Input: part model. Units: mm. Frame: model coordinates. Face numbers are marked on the shaded views. A direction names the side the tool comes from. Round coordinates to 2 decimals unless told otherwise and drop trailing zeros. Order: outer loops, then holes, each group sorted by start corner. A loop starts at its lowest first (then second) coordinate and runs counter-clockwise, first axis right, second up. Notation, with made-up numbers: (-29, 41) -> (10, 41) arc R20 cw to (10, 60) -> close; hole circle Ø11 at (-35, -20). An arc over 180 degrees is marked (long way). Answer as CSV lines item,"result". Start each with the question number.
1) Section query D-D, the plane y = -3.5. Output: boundary loops of the cut face in (x, z), and give its area (3 significant figures).
2) Line query: L1, parallel to Y at x = 10, z = 3.35; L2, parallel to X at y = 3.5, z = 3.25; L3, parallel to Y at x = 90.5, z = 1.5. Output: solid intervals per line, ascending.
3) Section query C-C, the plane z = 3.25. Output: boundary loops of the cut face in (x, y).
4) Section query B-B, the plane x = 10. Output: boundary loops of the cut face in (y, z).
5) Section query A-A, the plane y = 5. Output: boundary loops of the cut face in (x, z), and give its area (3 significant figures).
6) First-contact query: P1, Ø1, axis at y = 3.5, z = 3.5, coming from the +X side; P2, Ø1, axis at x = 36.5, z = 6, coming from the +Y side; P3, Ø1.6, axis at y = -1.5, z = 8.5, coming from the -X side; P4, Ø5, axis at x = 25, y = 5, coming from the +Z side. Flat tips, straight axial feed; report the tip coordinate or a pass-through.
7) Access query for the marked faces 1, 2 and 3. Directions: +Z, -Z, +X, -X, +Y, -Y. A direction counts if a zero-diameter tool reaches every point of the face in a straight line with its end or side. Return the directions, or none.
```python
from build123d import *

# Parameters (mm, degrees)
SKETCH_1_W          = 100
SKETCH_1_H          = 25
EXTRUDE_1_DEPTH     = 5
SKETCH_2_W          = 53
SKETCH_2_H          = 5
EXTRUDE_2_DEPTH     = 5
SKETCH_5_W          = 56
SKETCH_5_H          = 5
CUT_EXTRUDE_1_DEPTH = 10
SKETCH_6_W          = 5
SKETCH_6_H          = 5
EXTRUDE_3_DEPTH     = 47
SKETCH_7_W          = 56
SKETCH_7_H          = 5
CUT_EXTRUDE_2_DEPTH = 14.5
SKETCH_8_W          = 53
SKETCH_8_H          = 5.5
EXTRUDE_4_DEPTH     = 5.95
SKETCH_9_W          = 10.95
SKETCH_9_H          = 5.5
EXTRUDE_5_DEPTH     = 32.46
SKETCH_11_W         = 44
SKETCH_11_H         = 5
CUT_EXTRUDE_3_DEPTH = 15
SKETCH_12_R         = 2.25
CUT_EXTRUDE_4_DEPTH = 15


with BuildPart() as part:
    # 草图1 → 凸台-拉伸1 (new body)
    with BuildSketch(Plane.XY):
        with Locations((50, 12.5)):
            Rectangle(SKETCH_1_W, SKETCH_1_H)
    extrude(amount=EXTRUDE_1_DEPTH)

    # 草图2 → 凸台-拉伸2 (add)
    with BuildSketch(Plane.XZ):
        with Locations((73.5, 2.5)):
            Rectangle(SKETCH_2_W, SKETCH_2_H)
    extrude(amount=EXTRUDE_2_DEPTH)

    # 草图5 → 切除-拉伸1 (cut)
    with BuildSketch(Plane(origin=(0, 25, 0), x_dir=(1, 0, 0), z_dir=(0, 1, 0))):
        with Locations((72, -2.5)):
            Rectangle(SKETCH_5_W, SKETCH_5_H)
    extrude(amount=-CUT_EXTRUDE_1_DEPTH, mode=Mode.SUBTRACT)

    # 草图6 → 凸台-拉伸3 (add)
    with BuildSketch(Plane.ZY.offset(-47)):
        with Locations((2.5, -2.5)):
            Rectangle(SKETCH_6_W, SKETCH_6_H)
    extrude(amount=EXTRUDE_3_DEPTH)

    # 草图7 → 切除-拉伸2 (cut)
    with BuildSketch(Plane(origin=(0, 15, 0), x_dir=(1, 0, 0), z_dir=(0, 1, 0))):
        with Locations((72, -2.5)):
            Rectangle(SKETCH_7_W, SKETCH_7_H)
    extrude(amount=-CUT_EXTRUDE_2_DEPTH, mode=Mode.SUBTRACT)

    # 草图8 → 凸台-拉伸4 (add)
    with BuildSketch(Plane.XY.offset(5)):
        with Locations((73.5, -2.25)):
            Rectangle(SKETCH_8_W, SKETCH_8_H)
    extrude(amount=EXTRUDE_4_DEPTH)

    # 草图9 → 凸台-拉伸5 (add)
    with BuildSketch(Plane(origin=(100, 0, 0), x_dir=(0, 0, -1), z_dir=(1, 0, 0))):
        with Locations((-5.475, -2.25)):
            Rectangle(SKETCH_9_W, SKETCH_9_H)
    extrude(amount=EXTRUDE_5_DEPTH)

    # 草图11 → 切除-拉伸3 (cut)
    with BuildSketch(Plane(origin=(0, 25, 0), x_dir=(1, 0, 0), z_dir=(0, 1, 0))):
        with Locations((22, -2.5)):
            Rectangle(SKETCH_11_W, SKETCH_11_H)
    extrude(amount=-CUT_EXTRUDE_3_DEPTH, mode=Mode.SUBTRACT)

    # 草图12 → 切除-拉伸4 (cut)
    with BuildSketch(Plane(origin=(0, 0, 0), x_dir=(-1, 0, 0), z_dir=(0, 0, -1))):
        with Locations((-10, 5)):
            Circle(SKETCH_12_R)
        with Locations((-25, 5)):
            Circle(SKETCH_12_R)
    extrude(amount=-CUT_EXTRUDE_4_DEPTH, mode=Mode.SUBTRACT)


solid = part.part
```
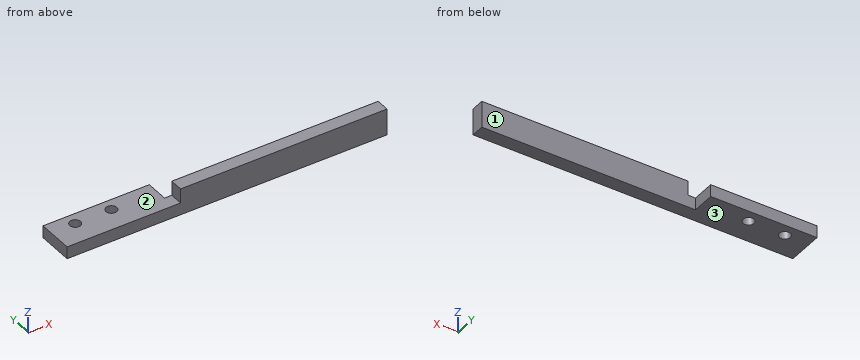
Findings:
1,outline,"(0, 0) -> (132.46, 0) -> (132.46, 10.95) -> (47, 10.95) -> (47, 5) -> (0, 5) -> close"
1,area,"1,170 mm^2"
2,L1,"y = -5 to 2.75, 7.25 to 10"
2,L2,"x = 0 to 8.32, 11.68 to 23.32, 26.68 to 44"
2,L3,"y = -5 to 0.5"
3,outline,"(0, -5) -> (132.46, -5) -> (132.46, 0.5) -> (44, 0.5) -> (44, 10) -> (0, 10) -> close; hole circle Ø4.5 at (10, 5); hole circle Ø4.5 at (25, 5)"
4,outline,"(-5, 0) -> (2.75, 0) -> (2.75, 5) -> (-5, 5) -> close; (7.25, 0) -> (10, 0) -> (10, 5) -> (7.25, 5) -> close"
5,outline,"(0, 0) -> (7.75, 0) -> (7.75, 5) -> (0, 5) -> close; (12.25, 0) -> (22.75, 0) -> (22.75, 5) -> (12.25, 5) -> close; (27.25, 0) -> (44, 0) -> (44, 5) -> (27.25, 5) -> close"
5,area,"175 mm^2"
6,P1,"stops at x = 44"
6,P2,"passes through"
6,P3,"stops at x = 47"
6,P4,"stops at z = 5"
7,face 1,"+Z, -Z, +X, +Y"
7,face 2,"+Z, -X, +Y, -Y"
7,face 3,"-Z, +X, -X, +Y, -Y"
